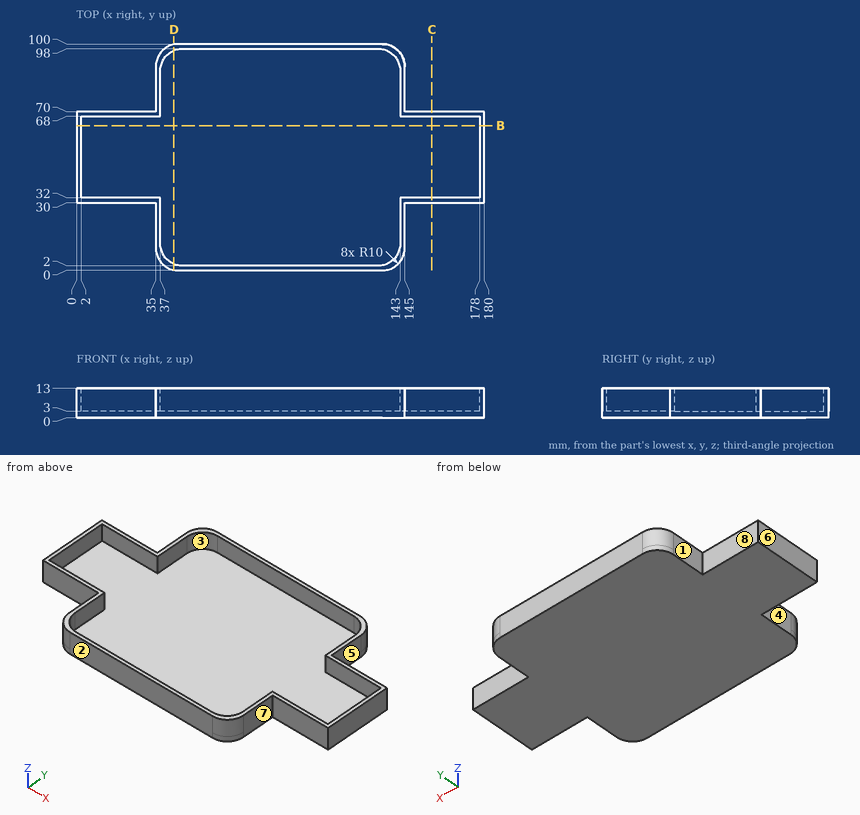
Source: three-view drawing plus pictorial views. Frame: mm from the lowest corner of the part. A direction names the side the tool comes from. Give positions to 0.01 mm unless a question says otherwise; leave off trailing zeros. Order: outer loops, then holes, each group sorted by start corner. A loop starts at its lowest first (then second) coordinate and runs counter-clockwise, first axis right, second up. Notation, with made-up numbers: M 78.5,16 L 116.5,16 A10 ccw 116.5,29 Z; hole C 36.5,20.25 d11. An arc over 180 degrees is marked long. Return JSON: item names as keys, results as strings.
1) Line query: L1, parallel to Y at x = 32.5, z = 4.5; L2, parallel to X at y = 75, z = 9; L3, parallel to Y at x = 90.5, z = 4.5. Output: solid intervals per line, ascending. Write a range as [from, to].
Taken from the geometry:
{"L1": "y = [30, 32], [68, 70]", "L2": "x = [35, 37], [143, 145]", "L3": "y = [0, 2], [98, 100]"}
2) Access query for the marked faces 4, 5, 6, 7 and 8. Directions: +Z, -Z, +X, -X, +Y, -Y. A direction counts if a zero-diameter tool reaches every point of the face in a straight line with its end or side. Return the directions, or none.
Taken from the geometry:
{"face 4": "+Z, -Z, -X, -Y", "face 5": "+Z, -Z, +X, +Y", "face 6": "+Z, -Z, -X, +Y, -Y", "face 7": "+Z, -Z, +X, -Y", "face 8": "+Z, -Z, -X, +Y"}
3) Section query B-B on y = 64. Output: boundary loops of the cut face in (x, z), and give its area (3 significant figures).
Taken from the geometry:
{"outline": "M 0,0 L 180,0 L 180,13 L 178,13 L 178,3 L 2,3 L 2,13 L 0,13 Z", "area": "580 mm2"}
4) Section query C-C on x = 157. Output: boundary loops of the cut face in (y, z), and give its area (3 significant figures).
Taken from the geometry:
{"outline": "M 30,0 L 70,0 L 70,13 L 68,13 L 68,3 L 32,3 L 32,13 L 30,13 Z", "area": "160 mm2"}
5) Section query D-D on x = 43. Output: boundary loops of the cut face in (y, z), and give its area (3 significant figures).
Taken from the geometry:
{"outline": "M 0.2,0 L 99.8,0 L 99.8,13 L 97.17,13 L 97.17,3 L 2.83,3 L 2.83,13 L 0.2,13 Z", "area": "351 mm2"}
6) Contact query for flat-ended pins moving along their axis: pin 1 (1.5 mm diameter, centred on x = 160, z = 7, fed in from +Y); pin 2 (3 mm diameter, centred on y = 26.5, z = 8.5, fed in from -X); pin 3 (3 mm diameter, centred on y = 80.5, z = 8, fed in from +X); pin 4 (5 mm diameter, centred on x = 48.5, y = 15, fed in from -Z). Output: stop coordinate, or through.
Taken from the geometry:
{"pin 1": "stops at y = 70", "pin 2": "stops at x = 35", "pin 3": "stops at x = 145", "pin 4": "stops at z = 0"}
7) Mould query, pull axis Y, two halves, no side actions, for the marked faces 1, 2 and 3. Classes: released by +Y, released by -Y, zero draft, split by the parting line, or undercut.
Taken from the geometry:
{"face 1": "zero draft", "face 2": "released by -Y", "face 3": "undercut"}
